Input: part model. Units: mm. Frame: model coordinates. A direction names the side the tool comes from. Give positions to 0.01 mm unless a question says otherwise; leave off trailing zeros. Answer in a Markdown table with one row per item. Add a question column.
1. Ray query, line 1 (X direction, y = -6.5, z = -5.5); line 2 (Z direction, x = 24, y = -3); line 3 (Z direction, x = 22.5, y = 0). Return the intervals inside material, ascending. Write a range as [from, to].
2. Contact query for flat-ended pins moving along their axis: pin 1 (2 mm diameter, centred on x = 27, y = 4, fed in from -Z); pin 2 (5 mm diameter, centred on y = -3.5, z = -7.5, fed in from +X); pin 3 (6 mm diameter, centred on x = 28.5, y = 2, fed in from +Z). Output: stop coordinate, or through.
3. Access query for faces 1 (the face through (6.9, 5, -8)), 2 (the face through (54.653, -5.994, 0.264)), 3 (the face through (3, 0, 9)). Directions: +Z, -Z, +X, -X, +Y, -Y. A direction counts if a zero-diameter tool reaches every point of the face in a straight line with its end or side. Return the directions, or none.
```python
from build123d import *

# Parameters (mm, degrees)
BASEHEAD_DEPTH  = 7.5
BASEBODY_START  = 6.9
BASEBODY_DEPTH  = 0.6
HEADFILLET_R    = 0.6
THDSCHPAT_COUNT = 34
THDSCHPAT_PITCH = 1.713235294


# Read off the part's stored shape, not the designer's step: BearingFace, BaseBody
with BuildPart() as part:
    # Sketch1 → BaseHead (new body)
    with BuildSketch(Plane(origin=(0, 0, 0), x_dir=(0, 0, -1), z_dir=(1, 0, 0))):
        Polygon((9, 5.196152423), (9, -5.196152423), (0, -10.392304845), (-9, -5.196152423), (-9, 5.196152423), (0, 10.392304845), align=None)
    extrude(amount=BASEHEAD_DEPTH)

    # BearingFace outline → BearingFace (revolve)
    with BuildSketch(Plane.YX):
        Polygon((6, 7.5), (6, 66.536), (5.036, 67.5), (0, 67.5), (0, 7.5), align=None)
    revolve(axis=Axis((0, 0, 0), (1, 0, 0)))

    # Sketch3 → HeadChamfer (revolve, cut)
    with BuildSketch(Plane.XY, mode=Mode.PRIVATE) as headchamfer_sk:
        Polygon((0, 9), (3.690598923, 15.392304845), (3.690598923, 20.392304845), (-10, 20.392304845), (-10, 9), align=None)
    revolve(headchamfer_sk.sketch.rotate(Axis((0, 0, 0), (1, 0, 0)), 90), axis=Axis((0, 0, 0), (1, 0, 0)), mode=Mode.SUBTRACT)

    # BaseBody outline → BaseBody (cut)
    with BuildSketch(Plane.YZ.offset(BASEBODY_START)):
        with BuildLine():
            ThreePointArc((7.794228634, 4.5), (9, 0), (7.794228634, -4.499999999))
            Line((7.794228634, -4.499999999), (10.392304845, 0))
            Line((10.392304845, 0), (7.794228634, 4.5))
        make_face()
        with BuildLine():
            ThreePointArc((0, 9), (4.5, 7.794228634), (7.794228634, 4.5))
            Line((7.794228634, 4.5), (5.196152423, 9))
            Line((5.196152423, 9), (0, 9))
        make_face()
        with BuildLine():
            Line((5.196152423, -9), (7.794228634, -4.499999999))
            ThreePointArc((7.794228634, -4.499999999), (4.5, -7.794228634), (0, -9))
            Line((0, -9), (5.196152423, -9))
        make_face()
        with BuildLine():
            ThreePointArc((-7.794228634, 4.5), (-4.5, 7.794228634), (0, 9))
            Line((0, 9), (-5.196152423, 9))
            Line((-5.196152423, 9), (-7.794228634, 4.5))
        make_face()
        with BuildLine():
            Line((-5.196152423, -9), (0, -9))
            ThreePointArc((0, -9), (-4.5, -7.794228634), (-7.794228634, -4.5))
            Line((-7.794228634, -4.5), (-5.196152423, -9))
        make_face()
        with BuildLine():
            ThreePointArc((-7.794228634, -4.5), (-9, 0), (-7.794228634, 4.5))
            Line((-7.794228634, 4.5), (-10.392304845, 0))
            Line((-10.392304845, 0), (-7.794228634, -4.5))
        make_face()
    extrude(amount=BASEBODY_DEPTH, mode=Mode.SUBTRACT)

    # HeadFillet
    headfillet_edges = [part.edges().sort_by_distance(p)[0] for p in [
        (7.5, -6, 0),
    ]]
    fillet(headfillet_edges, radius=HEADFILLET_R)

    # ThdSchSke → ThreadSchematic (revolve, cut)
    with BuildSketch(Plane.XY):
        Polygon((9.25, -5.036), (8.574999933, -6), (8.574999933, -7.5), (9.925000067, -7.5), (9.925000067, -6), align=None)
    threadschematic = revolve(axis=Axis((-3.175, 0, 0), (1, 0, 0)), mode=Mode.SUBTRACT)

    # ThdSchPat: ThreadSchematic ×34
    with Locations(*[(i * THDSCHPAT_PITCH, 0, 0) for i in range(1, THDSCHPAT_COUNT)]):
        add(threadschematic, mode=Mode.SUBTRACT)


solid = part.part
```
Answer:
| question | item | result |
|---|---|---|
| 1 | line 1 | x = [0, 7.5] |
| 1 | line 2 | z = [-5.19, 5.19] |
| 1 | line 3 | z = [-5.69, 5.69] |
| 2 | pin 1 | stops at z = -5.2 |
| 2 | pin 2 | stops at x = 66.76 |
| 2 | pin 3 | stops at z = 6 |
| 3 | face 1 | -Z, +X, +Y |
| 3 | face 2 | +X |
| 3 | face 3 | +Z, +X, -X, +Y, -Y |
